```python
from build123d import *

# Parameters (mm, degrees)
F0_R     = 54.7615085619
F0_R_2   = 19.9782226064
F1_DEPTH = 25.4
F2_W     = 14.4728478044
F2_H     = 5.7084001601
F3_DEPTH = 25.4
F4_R     = 0.508
F5_SIZE  = 5.08


# Not quite as in the source:
# - a fillet or chamfer that OpenCascade refuses, or shapes differently, is made with other operations: its cross-section is extruded or revolved along the edge and cut away or added


with BuildPart() as f1:
    # F0 (on Front) → F1 (new body)
    with BuildSketch(Plane.XZ):
        with Locations((-1.2108273804, -0.5243010819)):
            Circle(F0_R)
        with Locations((-0.7577873766, 2.7753412724)):
            Circle(F0_R_2, mode=Mode.SUBTRACT)
    extrude(amount=F1_DEPTH)

    # F2 (on face) → F3 (cut)
    with BuildSketch(Plane.XZ.offset(25.4)):
        with Locations((-10.4092946276, 42.7569095045)):
            Rectangle(F2_W, F2_H)
    extrude(amount=-F3_DEPTH, mode=Mode.SUBTRACT)

    # F4
    f4_edges = [f1.edges().sort_by_distance(p)[0] for p in [
        (-55.972336, -25.4, -0.524301),
    ]]
    fillet(f4_edges, radius=F4_R)

    # F5
    f5_edges = [f1.edges().sort_by_distance(p)[0] for p in [
        (-20.73601, -25.4, 2.775341),
    ]]
    chamfer(f5_edges, length=F5_SIZE)

    # F6: fillet of radius 16.8651706448 on 1 edges, made by hand

    # F6_s1 → F6_t2 (revolve, cut)
    with BuildSketch(Plane.XY.offset(-0.5243010819)):
        with BuildLine():
            ThreePointArc((53.5506811815, -16.8651706448), (48.6109870655, -4.939694116), (36.6855105367, 0))
            Line((36.6855105367, 0), (53.5506811815, 0))
            Line((53.5506811815, 0), (53.5506811815, -16.8651706448))
        make_face()
    revolve(axis=Axis((-1.2108273804, 0, -0.5243010819), (0, -1, 0)), mode=Mode.SUBTRACT)


solid = f1.part
```
Geometry: final body of the model. Coordinates: model frame, mm. A direction names the side the tool comes from. Give positions to 0.01 mm unless a question says otherwise; leave off trailing zeros. Write each loop counter-clockwise with the first axis right and the second up, starting at its lowest first coordinate (ties: lowest second). Pieces come first, ordered by that corner, then holes.
1. Section query B-B, the plane x = -11. Count the separate pieces of the cut face and the enclosed holes in it, then the cut area to 3 significant figures.
2. Section query C-C, the plane y = -5.5. Return loops of the section in (x, z), then the cut area to 3 significant figures.
3. Pin query (flat end, axial travel): P1, Ø1, axis at x = -9, y = -16.5, coming from the +Z side; P2, Ø10, axis at x = 39.5, y = -16, coming from the -Z side; P3, Ø4, axis at x = -33.5, y = -13, coming from the -Z side. Return the tip coordinate at first contact, or that it passes through.
4. Line query: probe 1 along X at (y, z) = (-6, -5); probe 2 along Z at (x, y) = (-15, -13); probe 3 along X at (y, z) = (-16, -12.5). Output: solid intervals per line, ascending.
5. Section query A-A, the plane y = -12.5. Return loops of the section in (x, z).
6. Draft query along X for faces 1 (the cylindrical face through (-20.717, -10.018, 3.654)), 2 (the conical face through (18.533, -20.567, 8.85)), 3 (the cylindrical face through (-13, -21, -54)), 4 (the flat face through (-2, -25.4, -24)). Return one class per face: released by +X, released by -X, zero draft, split by the parting line, or undercut.
7. Reachability of faces 5 (the flat face through (7, 0, -17)), 6 (the flat face through (-3.173, -13, 43)) from +Z, -Z, +X, -X, +Y, -Y: full face, straight path, thin tool, end or side. Return the list, or none.
Computed:
1. separate pieces: 3
1. enclosed holes: 0
1. area: 1,570 mm2
2. outline: circle Ø100.71 at (-1.21, -0.52); hole circle Ø39.96 at (-0.76, 2.78); hole (-17.65, 39.9) - (-3.17, 39.9) - (-3.17, 45.61) - (-17.65, 45.61) - close
2. area: 6,630 mm2
3. P1: stops at z = 53.75
3. P2: stops at z = -42.02
3. P3: stops at z = -45.7
4. probe 1: x = -51.81 to -19.16, 17.65 to 49.39
4. probe 2: z = -53.06 to -11.23, 16.79 to 39.9, 45.61 to 52.01
4. probe 3: x = -54.62 to -13.63, 12.12 to 52.2
5. outline: circle Ø108.37 at (-1.21, -0.52); hole circle Ø39.96 at (-0.76, 2.78); hole (-17.65, 39.9) - (-3.17, 39.9) - (-3.17, 45.61) - (-17.65, 45.61) - close
6. face 1: undercut
6. face 2: undercut
6. face 3: split by the parting line
6. face 4: zero draft
7. face 5: +Z, -Z, +X, -X, +Y
7. face 6: +Y, -Y
